Autodesk Inventor part; units mm, degrees
ref_plane "YZ Plane" through (0, 0, 0) normal (1, 0, 0) x (0, 1, 0)
ref_plane "XZ Plane" through (0, 0, 0) normal (0, 1, 0) x (-1, 0, 0)
ref_plane "XY Plane" through (0, 0, 0) normal (0, 0, 1) x (1, 0, 0)
sketch "スケッチ1" plane through (0, 0, 0) normal (0, 0, 1) x (1, 0, 0)
  line L0 (0, 0) -> (8, 0)
  line L1 (8, 0) -> (8, -8)
  line L2 (8, -8) -> (0, -8)
  line L3 (0, -8) -> (0, 0)
  line L4 (0, -4) -> (8, -4)
  line L5 (4, 0) -> (4, -8)
  dimension "d0" = 8
  dimension "d1" = 8
extrude "押し出し1" add sketch "スケッチ1" along normal blind 8
sketch "スケッチ2" plane through (8, -8, 0) normal (1, 0, 0) x (0, 0, -1)
  line L0 (-8, 8) -> (0, 8)
  line L1 (0, 8) -> (0, 0)
  line L2 (0, 0) -> (-8, 0)
  line L3 (-8, 0) -> (-8, 8)
  line L4 (-8, 8) -> (0, 0)
  line L5 (0, 8) -> (0, 0)
  line L6 (-8, 0) -> (0, 8)
  point P0 (-4, 4)
hole "穴1" at (8, -4, 4) direction (-1, 0, 0) diameter 2.5 end through all
sketch "スケッチ3" plane through (0, 0, 0) normal (0, 1, 0) x (1, 0, 0)
  line L0 (8, 0) -> (8, -8)
  line L1 (8, -8) -> (0, -8)
  line L2 (0, -8) -> (0, 0)
  line L3 (0, 0) -> (8, 0)
  line L4 (0, -8) -> (8, 0)
  line L5 (8, 0) -> (8, -8)
  line L6 (0, 0) -> (8, 0)
  line L7 (8, -8) -> (0, 0)
  point P0 (4, -4)
hole "穴2" at (4, 0, 4) direction (0, -1, 0) diameter 2.5 end through all
equation "\"d0\" = d1"
properties part number "垂直ブロック 真鍮 8" material "真鍮、ソフト イエロー"
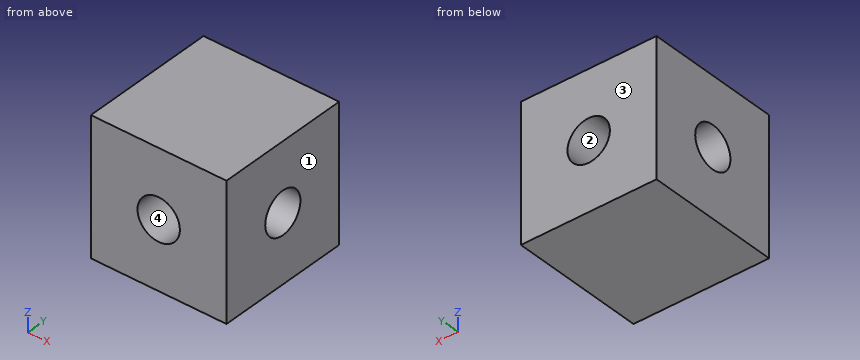
For this review, take the finished solid that the model builds, in its own axes (mm). Face numbers are marked on the shaded views. Round coordinates to 2 decimals unless told otherwise and drop trailing zeros. Write each loop counter-clockwise with the first axis right and the second up, starting at its lowest first coordinate (ties: lowest second). Pieces come first, ordered by that corner, then holes. Notation, with made-up numbers: (51.5, -25.75) - (56.5, -25.75) arc R24 cw to (56.5, 13.25) - close; hole circle Ø8 at (-11, -34). An arc over 180 degrees is marked (long way). Write item = value, one per line. Start each with the question number.
1. Consider section A-A on z = 3.25. State the section outline as (x, y) points.
2. Consider section C-C on y = -5.75. State the section outline as (x, z) points.
3. Draft analysis for pull direction X (two halves, no side actions). For the marked faces 1, 2, 3 and 4, state which applies: released by +X, released by -X, zero draft, split by the parting line, or undercut.
4. Wall thickness on L1, parallel to Z at x = 4, y = -5.1; L2, parallel to Y at x = 6.25, z = 4: over which ranges is each line inside the solid? List them lowest first.
5. Consider section D-D on x = 5.5. State the section outline as (y, z) points.
6. Consider section B-B on x = 4.5. State the section outline as (y, z) points, plus the area to 3 significant figures.
Evaluation:
q1.outline = (0, -8) - (3, -8) - (3, -5) - (0, -5) - close; (0, -3) - (3, -3) - (3, 0) - (0, 0) - close; (5, -8) - (8, -8) - (8, -5) - (5, -5) - close; (5, -3) - (8, -3) - (8, 0) - (5, 0) - close
q2.outline = (0, 0) - (8, 0) - (8, 8) - (0, 8) - close; hole circle Ø2.5 at (4, 4)
q3.face_1 = released by +X
q3.face_2 = undercut
q3.face_3 = zero draft
q3.face_4 = undercut
q4.L1 = 0 to 2.75, 5.25 to 8
q4.L2 = -8 to -5.25, -2.75 to 0
q5.outline = (-8, 0) - (0, 0) - (0, 8) - (-8, 8) - close; hole circle Ø2.5 at (-4, 4)
q6.outline = (-8, 0) - (0, 0) - (0, 2.85) - (-3.5, 2.85) arc R1.25 cw to (-4.5, 2.85) - (-8, 2.85) - close; (-8, 5.15) - (-4.5, 5.15) arc R1.25 cw to (-3.5, 5.15) - (0, 5.15) - (0, 8) - (-8, 8) - close
q6.area = 45.5 mm2
